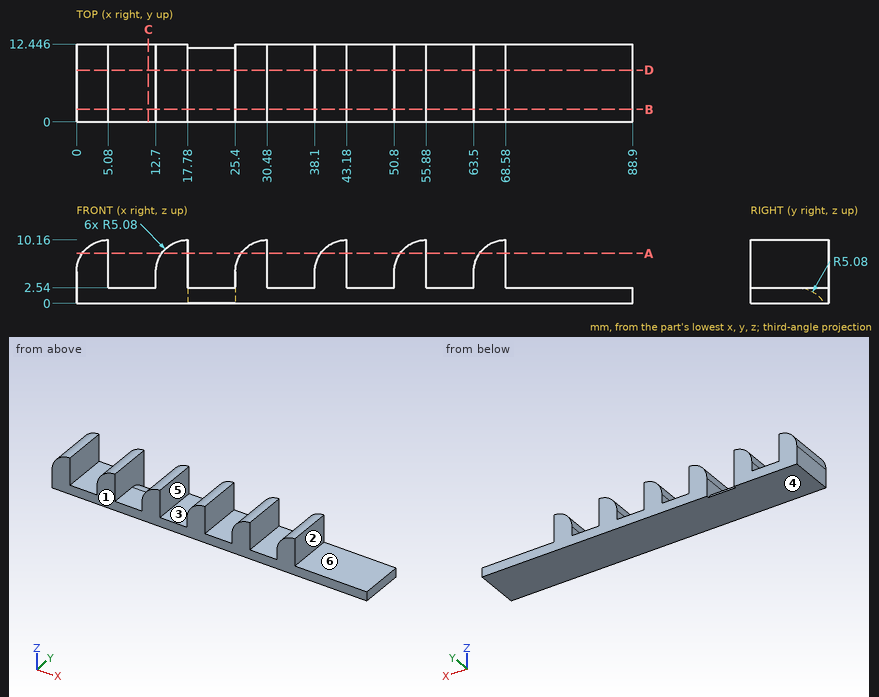
Input: dimensioned drawing with shaded views. Units: mm. Origin: part minimum x, y, z. A direction names the side the tool comes from. Round coordinates to 2 decimals unless told otherwise and drop trailing zeros. Order: outer loops, then holes, each group sorted by start corner. A loop starts at its lowest first (then second) coordinate and runs counter-clockwise, first axis right, second up. Notation, with made-up numbers: M 55,39.5 L 85,39.5 A36 ccw 85,75.5 Z; hole C 44.5,2 d4. An arc over 180 degrees is marked long. Use one line per item in the form item = value. Start each with the question number.
Q1. Cut plane C-C (x = 11.5). Return loops of the section in (y, z).
Q2. Material intervals for line 1 (X direction, y = 5.25, z = 3.25); line 2 (X direction, y = 1, z = 6.75); line 3 (Z direction, x = 75.5, y = 3.5), sorted ascending. Write a range as [from, to].
Q3. Pin query (flat end, axial travel): pin 1 Ø6 at (y, z) = (8, 6.5) entering from +X; pin 2 Ø6 at (x, y) = (61.5, 8.5) entering from +Z; pin 3 Ø5 at (x, y) = (26.5, 11) entering from +Z. Return the tip coordinate at first contact, or that it passes through.
Q4. Cut plane D-D (y = 8.25). Return loops of the section in (x, z).
Q5. Mould query, pull axis X, two halves, no side actions, for the marked faces 1, 2 and 3. Classes: +X half, -X half, draft (parallel to the pull), parting line (faces both ways), or undercut.
Q6. Cut plane A-A (z = 8). Return loops of the section in (x, y), and give its area (3 significant figures).
Q7. Cut plane B-B (y = 2). Return loops of the section in (x, z), and give its area (3 significant figures).
Q8. Access query for the marked faces 4, 5 and 6. Directions: +Z, -Z, +X, -X, +Y, -Y. A direction counts if a zero-diameter tool reaches every point of the face in a straight line with its end or side. Return the directions, or none.
Geometry results:
q1.outline = M 0,0 L 12.45,0 L 12.45,2.54 L 0,2.54 Z
q2.line_1 = [0, 5.08], [12.7, 17.78], [25.4, 30.48], [38.1, 43.18], [50.8, 55.88], [63.5, 68.58]
q2.line_2 = [0.28, 5.08], [12.98, 17.78], [25.68, 30.48], [38.38, 43.18], [51.08, 55.88], [63.78, 68.58]
q2.line_3 = [0, 2.54]
q3.pin_1 = 68.58
q3.pin_2 = 8.11
q3.pin_3 = 9.94
q4.outline = M 0,0 L 88.9,0 L 88.9,2.54 L 68.58,2.54 L 68.58,10.16 A5.08 ccw 63.5,5.08 L 63.5,2.54 L 55.88,2.54 L 55.88,10.16 A5.08 ccw 50.8,5.08 L 50.8,2.54 L 43.18,2.54 L 43.18,10.16 A5.08 ccw 38.1,5.08 L 38.1,2.54 L 30.48,2.54 L 30.48,10.16 A5.08 ccw 25.4,5.08 L 25.4,2.46 L 17.78,2.46 L 17.78,10.16 A5.08 ccw 12.7,5.08 L 12.7,2.54 L 5.08,2.54 L 5.08,10.16 A5.08 ccw 0,5.08 Z
q5.face_1 = draft
q5.face_2 = +X half
q5.face_3 = undercut
q6.outline = M 0.92,0 L 5.08,0 L 5.08,12.45 L 0.92,12.45 Z; M 13.62,0 L 17.78,0 L 17.78,12.45 L 13.62,12.45 Z; M 26.32,0 L 30.48,0 L 30.48,12.45 L 26.32,12.45 Z; M 39.02,0 L 43.18,0 L 43.18,12.45 L 39.02,12.45 Z; M 51.72,0 L 55.88,0 L 55.88,12.45 L 51.72,12.45 Z; M 64.42,0 L 68.58,0 L 68.58,12.45 L 64.42,12.45 Z
q6.area = 310 mm^2
q7.outline = M 0,0 L 88.9,0 L 88.9,2.54 L 68.58,2.54 L 68.58,10.16 A5.08 ccw 63.5,5.08 L 63.5,2.54 L 55.88,2.54 L 55.88,10.16 A5.08 ccw 50.8,5.08 L 50.8,2.54 L 43.18,2.54 L 43.18,10.16 A5.08 ccw 38.1,5.08 L 38.1,2.54 L 30.48,2.54 L 30.48,10.16 A5.08 ccw 25.4,5.08 L 25.4,2.54 L 17.78,2.54 L 17.78,10.16 A5.08 ccw 12.7,5.08 L 12.7,2.54 L 5.08,2.54 L 5.08,10.16 A5.08 ccw 0,5.08 Z
q7.area = 425 mm^2
q8.face_4 = -Z, +X, -X, +Y, -Y
q8.face_5 = +Z, +Y, -Y
q8.face_6 = +Z, +X, +Y, -Y
